For this review, take the finished solid that the model builds, in its own axes (mm). Face numbers are marked on the shaded views. A direction names the side the tool comes from. Round coordinates to 2 decimals unless told otherwise and drop trailing zeros. Loops run counter-clockwise (first coordinate to the right, second up) from the corner with the lowest first, then second, coordinate; pieces in that order, holes last.
1. Draft analysis for pull direction X (two halves, no side actions). For the marked faces 1, 2 and 3, state which applies: released by +X, released by -X, zero draft, split by the parting line, or undercut.
2. Clearance check with a flat-ended pin moving along its axis: pin 1 Ø4 at (x, y) = (45, -7.5) entering from -Z. State where the tip first meets the part, or that it passes through.
3. Tool access review of the marked faces 4 and 5: name each direction out of +Z, -Z, +X, -X, +Y, -Y from which nothing blocks a thin tool from reaching the whole face with its end or side.
4. Consider section A-A on z = 15.5. State the section outline as (x, y) points.
5. Consider section B-B on x = 29.5. State the section outline as (y, z) points.
6. Consider section C-C on x = 85. State the section outline as (y, z) points.
7. To check wall thickness, follow line 1 along X through (y, z) = (-4.5, 12); line 2 along X through (y, z) = (8.75, 14); line 3 along Y through (x, z) = (73.45, 11.2). State the ranges of each line that lie inside material, in increasing order.
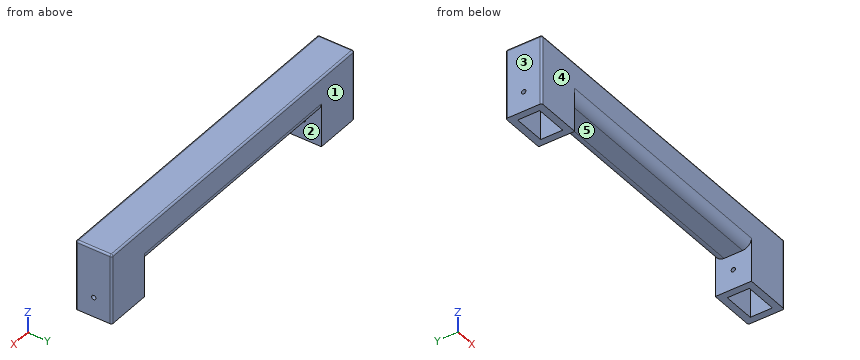
from build123d import *

# Parameters (mm, degrees)
F0_W     = 26.5
F0_H     = 20.6
F0_W_2   = 18.5
F0_H_2   = 12.6
F1_DEPTH = 20
F2_W     = 195
F2_H     = 20.6
F3_DEPTH = 20
F4_R     = 1
F5_R     = 1.25
F6_DEPTH = 2000
F7_R     = 1.25
F8_DEPTH = 100
F9_R     = 5


with BuildPart() as f1:
    # F0 (on Top) → F1 (new body)
    with BuildSketch(Plane.XY):
        with Locations((-84.25, 0)):
            Rectangle(F0_W, F0_H)
        with Locations((-84.25, 0)):
            Rectangle(F0_W_2, F0_H_2, mode=Mode.SUBTRACT)
    extrude(amount=F1_DEPTH)



with BuildPart() as f1b:
    # F0 (on Top) → F1, piece 2 (new body)
    with BuildSketch(Plane.XY):
        with Locations((84.25, 0)):
            Rectangle(F0_W, F0_H)
        with Locations((84.25, 0)):
            Rectangle(F0_W_2, F0_H_2, mode=Mode.SUBTRACT)
    extrude(amount=F1_DEPTH)


with BuildPart() as f1_1:
    add(f1.part)

    add(f1b.part)  # F3 merges F1b
    # F2 (on face) → F3 (join)
    with BuildSketch(Plane.XY.offset(20)):
        Rectangle(F2_W, F2_H)
    extrude(amount=F3_DEPTH)

    # F4
    f4_edges = [f1_1.edges().sort_by_distance(p)[0] for p in [
        (-97.5, 0, 40),
        (0, -10.3, 40),
        (97.5, 0, 40),
        (0, 10.3, 40),
        (-97.5, -10.3, 20),
        (97.5, -10.3, 20),
        (97.5, 10.3, 20),
        (-97.5, 10.3, 20),
    ]]
    fillet(f4_edges, radius=F4_R)

    # F5 (on face) → F6 (cut)
    with BuildSketch(Plane(origin=(-97.5, 0, 0), x_dir=(0, -1, 0), z_dir=(-1, 0, 0))):
        with Locations((0, 11.2)):
            Circle(F5_R)
    extrude(amount=-F6_DEPTH, mode=Mode.SUBTRACT)

    # F7 (on face) → F8 (cut)
    with BuildSketch(Plane.YZ.offset(97.5)):
        with Locations((0, 11.2)):
            Circle(F7_R)
    extrude(amount=-F8_DEPTH, mode=Mode.SUBTRACT)

    # F9
    f9_edges = [f1_1.edges().sort_by_distance(p)[0] for p in [
        (0, 10.3, 20),
        (0, -10.3, 20),
    ]]
    fillet(f9_edges, radius=F9_R)


solid = f1_1.part
Resolved:
1. face 1: zero draft
1. face 2: undercut
1. face 3: released by -X
2. pin 1: stops at z = 20
3. face 4: +Z, -Z, +X, -X, -Y
3. face 5: -Z, +Y, -Y
4. outline: (-97.5, -9.3) arc R1 ccw to (-96.5, -10.3) - (-71, -10.3) - (-71, 10.3) - (-96.5, 10.3) arc R1 ccw to (-97.5, 9.3) - close; (71, -10.3) - (96.5, -10.3) arc R1 ccw to (97.5, -9.3) - (97.5, 9.3) arc R1 ccw to (96.5, 10.3) - (71, 10.3) - close; hole (-93.5, -6.3) - (-75, -6.3) - (-75, 6.3) - (-93.5, 6.3) - close; hole (75, -6.3) - (93.5, -6.3) - (93.5, 6.3) - (75, 6.3) - close
5. outline: (-10.3, 25) arc R5 ccw to (-5.3, 20) - (5.3, 20) arc R5 ccw to (10.3, 25) - (10.3, 39) arc R1 ccw to (9.3, 40) - (-9.3, 40) arc R1 ccw to (-10.3, 39) - close
6. outline: (-10.3, 0) - (-6.3, 0) - (-6.3, 20) - (6.3, 20) - (6.3, 0) - (10.3, 0) - (10.3, 39) arc R1 ccw to (9.3, 40) - (-9.3, 40) arc R1 ccw to (-10.3, 39) - close
7. line 1: x = -97.5 to -93.5, -75 to -71, 71 to 75, 93.5 to 97.5
7. line 2: x = -97.5 to -71, 71 to 97.5
7. line 3: y = -10.3 to -1.25, 1.25 to 10.3
